```python
from build123d import *

# Parameters (mm, degrees)
SKETCH1_W           = 260
SKETCH1_H           = 200
BOSS_EXTRUDE1_DEPTH = 50
FILLET1_R           = 2
SHELL1_T            = -1
SKETCH2_W           = 41
SKETCH2_H           = 10
SKETCH2_W_2         = 18
SKETCH2_W_3         = 13
SKETCH2_H_2         = 5
SKETCH2_W_4         = 23
SKETCH2_W_5         = 20
SKETCH2_H_3         = 28
CUT_EXTRUDE1_DEPTH  = 50
SKETCH3_R           = 7.5
CUT_EXTRUDE2_DEPTH  = 50


with BuildPart() as part:
    # Sketch1 → Boss-Extrude1 (new body)
    with BuildSketch(Plane(origin=(0, 0, 0), x_dir=(1, 0, 0), z_dir=(0, 1, 0))):
        Rectangle(SKETCH1_W, SKETCH1_H)
    extrude(amount=BOSS_EXTRUDE1_DEPTH)

    # Fillet1
    fillet1_edges = [part.edges().sort_by_distance(p)[0] for p in [
        (0, 0, -100),
        (130, 0, 0),
        (0, 0, 100),
        (-130, 0, 0),
        (-130, 25, -100),
        (130, 25, -100),
        (130, 25, 100),
        (-130, 25, 100),
    ]]
    fillet(fillet1_edges, radius=FILLET1_R)

    # Shell1
    shell1_openings = [part.faces().sort_by_distance(p)[0] for p in [
        (0, 50, 0),
    ]]
    offset(amount=SHELL1_T, openings=shell1_openings, kind=Kind.INTERSECTION)

    # Sketch2 → Cut-Extrude1 (cut)
    with BuildSketch(Plane(origin=(130, 0, 0), x_dir=(0, 0, -1), z_dir=(1, 0, 0))):
        with Locations((-19, 15)):
            Rectangle(SKETCH2_W, SKETCH2_H)
        with Locations((-19, 35)):
            Rectangle(SKETCH2_W_2, SKETCH2_H)
        with Locations((26.5, 25)):
            Rectangle(SKETCH2_W_3, SKETCH2_H_2)
        with Locations((61.5, 25)):
            Rectangle(SKETCH2_W_4, SKETCH2_H_2)
        with Locations((-73, 25)):
            Rectangle(SKETCH2_W_5, SKETCH2_H_3)
    extrude(amount=-CUT_EXTRUDE1_DEPTH, mode=Mode.SUBTRACT)

    # Sketch3 → Cut-Extrude2 (cut)
    with BuildSketch(Plane.ZY.offset(130)):
        with Locations((58, 25)):
            Circle(SKETCH3_R)
    extrude(amount=-CUT_EXTRUDE2_DEPTH, mode=Mode.SUBTRACT)


solid = part.part
```
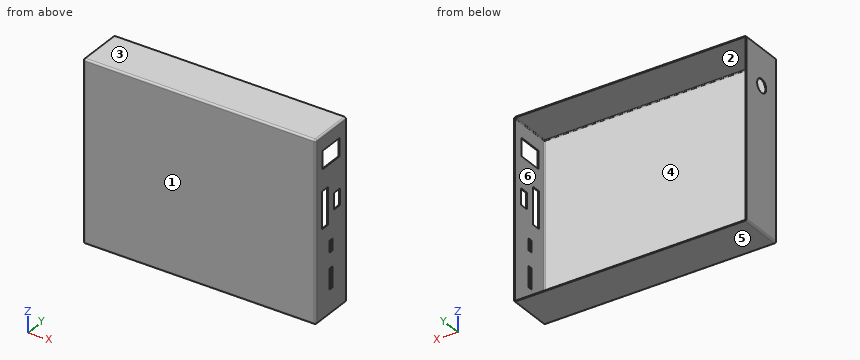
CAD build for the part. Positions are in the model's coordinates, mm. Face numbers are marked on the shaded views. A direction names the side the tool comes from. Coordinates: 2 decimals unless noted, no trailing zeros. Order: outer loops, then holes, each group sorted by start corner. A loop starts at its lowest first (then second) coordinate and runs counter-clockwise, first axis right, second up.
(1) Which spindle directions (+Z, -Z, +X, -X, +Y, -Y) get a long thin tool onto all of the face, cutting with end or side? Do the marked faces 5 and 6. Say none if no direction does.
Solution:
face 5: -Z, +X, -X, +Y, -Y
face 6: +Y
(2) Drill centre lines: L1, parallel to X at y = 27, z = 43.5; L2, parallel to Z at x = 77, y = 2.5; L3, parallel to Y at x = 5.5, z = 44.5. Where is each one in solid material? Low to high.
Solution:
L1: x = -130 to -129, 129 to 130
L2: z = -100 to -99, 99 to 100
L3: y = 0 to 1
(3) Saw through at A-A, the plane y = 14. Write the cut outline in (x, z).
Solution:
outline: (-130, -98) arc R2 ccw to (-128, -100) - (128, -100) arc R2 ccw to (130, -98) - (130, -1.5) - (129, -1.5) - (129, -98) arc R1 cw to (128, -99) - (-128, -99) arc R1 cw to (-129, -98) - (-129, 98) arc R1 cw to (-128, 99) - (128, 99) arc R1 cw to (129, 98) - (129, 83) - (130, 83) - (130, 98) arc R2 ccw to (128, 100) - (-128, 100) arc R2 ccw to (-130, 98) - close; (129, 39.5) - (130, 39.5) - (130, 63) - (129, 63) - close
(4) Saw through at D-D, the plane x = -44. Write the cut outline in (y, z), and give its area (3 significant figures).
Solution:
outline: (0, -98) arc R2 ccw to (2, -100) - (50, -100) - (50, -99) - (2, -99) arc R1 cw to (1, -98) - (1, 98) arc R1 cw to (2, 99) - (50, 99) - (50, 100) - (2, 100) arc R2 ccw to (0, 98) - close
area: 297 mm2
(5) Pin check, flat tips, straight feed: pin 1 Ø1 at (x, z) = (22.5, -13) entering from +Y; pin 2 Ø0.5 at (x, y) = (129.5, 35.5) entering from +Z; pin 3 Ø9 at (y, z) = (25, 58) entering from -X. Stop position of each tip, or through.
Solution:
pin 1: stops at y = 1
pin 2: stops at z = 99.56
pin 3: stops at x = 129
(6) Mould opens along Z. For the marked faces 1, 2, 3 and 4 say: released by +Z, released by -Z, zero draft, split by the parting line, or undercut.
Solution:
face 1: zero draft
face 2: undercut
face 3: released by +Z
face 4: undercut
(7) Saw through at C-C, the plane y = 43.5. Write the cut outline in (x, z).
Solution:
outline: (-130, -98) arc R2 ccw to (-128, -100) - (128, -100) arc R2 ccw to (130, -98) - (130, 98) arc R2 ccw to (128, 100) - (-128, 100) arc R2 ccw to (-130, 98) - close; hole (-129, -98) arc R1 ccw to (-128, -99) - (128, -99) arc R1 ccw to (129, -98) - (129, 98) arc R1 ccw to (128, 99) - (-128, 99) arc R1 ccw to (-129, 98) - close
(8) Saw through at B-B, the plane z = -56. Write the cut outline in (x, y), and give its area (3 significant figures).
Solution:
outline: (-130, 2) arc R2 ccw to (-128, 0) - (128, 0) arc R2 ccw to (130, 2) - (130, 22.5) - (129, 22.5) - (129, 2) arc R1 cw to (128, 1) - (-128, 1) arc R1 cw to (-129, 2) - (-129, 50) - (-130, 50) - close; (129, 27.5) - (130, 27.5) - (130, 50) - (129, 50) - close
area: 352 mm2
